Geometry: final body of the model. Coordinates: model frame, mm. Face numbers are marked on the shaded views. A direction names the side the tool comes from. Give positions to 0.01 mm unless a question says otherwise; leave off trailing zeros. Order: outer loops, then holes, each group sorted by start corner. A loop starts at its lowest first (then second) coordinate and runs counter-clockwise, first axis right, second up. Notation, with made-up numbers: (37.5, 76) - (82.5, 76) arc R25 cw to (82.5, 109) - close; hole circle Ø9 at (7.5, -4.75). An arc over 180 degrees is marked (long way). Use one line per item in the form item = value.
from build123d import *
from OCP.BRepFilletAPI import BRepFilletAPI_MakeChamfer

# Parameters (mm, degrees)
SKETCH1_W           = 12.7
SKETCH1_H           = 16
BOSS_EXTRUDE1_DEPTH = 22
SKETCH2_R           = 2.75
CUT_EXTRUDE1_DEPTH  = 239.308352823
SKETCH5_W           = 168.195
SKETCH5_H           = 59.75
CUT_EXTRUDE3_DEPTH  = 8
CHAMFER1_SIZE       = 10
CHAMFER1_SIZE2      = 5.773502692
SKETCH7_R           = 5.25
CUT_EXTRUDE4_DEPTH  = 10
CHAMFER2_SIZE       = 12


with BuildPart() as part:
    # Sketch1 → Boss-Extrude1 (new body)
    with BuildSketch(Plane.XY):
        Polygon((-12, 31.75), (200.195, 31.75), (233.895, 31.75), (233.895, -40), (200.895, -40), (-12.7, -40), (-45.7, -40), (-45.7, 31.75), align=None)
        with Locations((-6.35, -4.125)):
            Rectangle(SKETCH1_W, SKETCH1_H, mode=Mode.SUBTRACT)
        with Locations((194.545, -4.125)):
            Rectangle(SKETCH1_W, SKETCH1_H, mode=Mode.SUBTRACT)
    extrude(amount=BOSS_EXTRUDE1_DEPTH)

    # Sketch2 → Cut-Extrude1 (cut, through all)
    with BuildSketch(Plane.XY.offset(22)):
        with Locations((-6.35, 19.75)):
            Circle(SKETCH2_R)
        with Locations((-6.35, -28)):
            Circle(SKETCH2_R)
        with Locations(Location((194.545, -28, 0), (0, 0, 180))):
            Circle(SKETCH2_R)
        with Locations(Location((194.545, 19.75, 0), (0, 0, 180))):
            Circle(SKETCH2_R)
    extrude(amount=-CUT_EXTRUDE1_DEPTH, mode=Mode.SUBTRACT)

    # Sketch5 → Cut-Extrude3 (cut)
    with BuildSketch(Plane(origin=(0, 0, 0), x_dir=(-1, 0, 0), z_dir=(0, 0, -1))):
        with Locations((-94.0975, -10.125)):
            Rectangle(SKETCH5_W, SKETCH5_H)
    extrude(amount=-CUT_EXTRUDE3_DEPTH, mode=Mode.SUBTRACT)

    # Chamfer1: one chamfer whose edges measure the first distance from different faces: ONE call of the kernel's chamfer builder (chamfer() names one face for all edges)
    chamfer1_edges_1 = [part.edges().sort_by_distance(p)[0] for p in [
        (94.0975, -40, 22),
    ]]
    chamfer1_side_1 = [part.faces().sort_by_distance(p)[0] for p in [
        (94.0975, -40, 12.960016897),
    ]]
    chamfer1_edges_2 = [part.edges().sort_by_distance(p)[0] for p in [
        (94.0975, 31.75, 22),
    ]]
    chamfer1_side_2 = [part.faces().sort_by_distance(p)[0] for p in [
        (94.0975, 31.75, 11),
    ]]
    chamfer1 = BRepFilletAPI_MakeChamfer(part.part.solid().wrapped)
    for e in chamfer1_edges_1:
        chamfer1.Add(CHAMFER1_SIZE, CHAMFER1_SIZE2, e.wrapped, chamfer1_side_1[0].wrapped)  # the first distance lies on this face
    for e in chamfer1_edges_2:
        chamfer1.Add(CHAMFER1_SIZE, CHAMFER1_SIZE2, e.wrapped, chamfer1_side_2[0].wrapped)  # the first distance lies on this face
    add(Compound.cast(chamfer1.Shape()), mode=Mode.REPLACE)

    # Sketch7 → Cut-Extrude4 (cut)
    with BuildSketch(Plane.XY.offset(22)):
        with Locations((-6.35, 19.75)):
            Circle(SKETCH7_R)
        with Locations((-6.35, -28)):
            Circle(SKETCH7_R)
        with Locations((194.545, 19.75)):
            Circle(SKETCH7_R)
        with Locations((194.545, -28)):
            Circle(SKETCH7_R)
    extrude(amount=-CUT_EXTRUDE4_DEPTH, mode=Mode.SUBTRACT)

    # Chamfer2
    chamfer2_edges = [part.edges().sort_by_distance(p)[0] for p in [
        (-45.7, -4.125, 22),
        (233.895, -4.125, 22),
    ]]
    chamfer(chamfer2_edges, length=CHAMFER2_SIZE)


solid = part.part
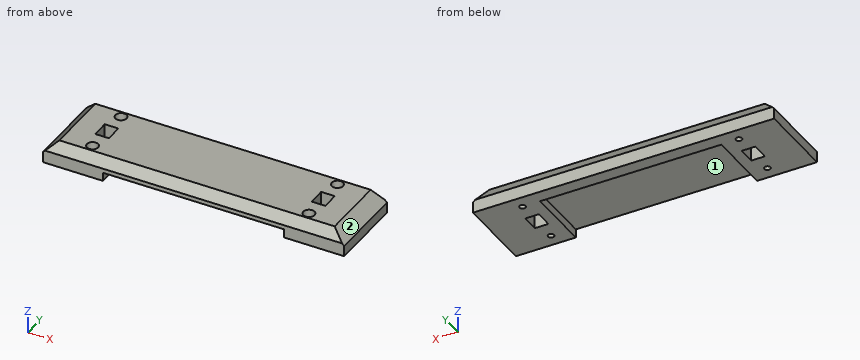
(1) Cut plane D-D on z = 5. Output: boundary loops of the cut face in (x, y) (3 decimals).
Computed values:
outline = (-45.7, -40) - (10, -40) - (10, 19.75) - (178.195, 19.75) - (178.195, -40) - (233.895, -40) - (233.895, 31.75) - (-45.7, 31.75) - close; hole (-12.7, -12.125) - (0, -12.125) - (0, 3.875) - (-12.7, 3.875) - close; hole circle Ø5.5 at (-6.35, -28); hole circle Ø5.5 at (-6.35, 19.75); hole (188.195, -12.125) - (200.895, -12.125) - (200.895, 3.875) - (188.195, 3.875) - close; hole circle Ø5.5 at (194.545, -28); hole circle Ø5.5 at (194.545, 19.75)
(2) Reachability of the marked faces 1 and 2 from +Z, -Z, +X, -X, +Y, -Y: full face, straight path, thin tool, end or side. Return the list, or none.
Computed values:
face_1 = -Z, -Y
face_2 = +Z, +X, +Y, -Y
(3) Cut plane B-B on x = 170. Output: boundary loops of the cut face in (y, z), plus the area to 3 significant figures.
Computed values:
outline = (-40, 8) - (19.75, 8) - (19.75, 0) - (31.75, 0) - (31.75, 12) - (25.98, 22) - (-34.23, 22) - (-40, 12) - close
area = 1,040 mm²
(4) Cut plane C-C on x = -6.35. Give the number of separate pieces and of enclosed holes in the cut face, plus the area to 3 significant figures.
Computed values:
separate_pieces = 4
enclosed_holes = 0
area = 827 mm²
(5) Contact query for flat-ended pins moving along their axis: pin 1 Ø4 at (x, y) = (126, -14) entering from -Z; pin 2 Ø6 at (x, z) = (96, 18.5) entering from -Y; pin 3 Ø8.5 at (x, y) = (194.545, -28) entering from +Z. Output: stop coordinate, or through.
Computed values:
pin_1 = 8
pin_2 = -37.98
pin_3 = 12
(6) Cut plane A-A on y = 1.5. Output: boundary loops of the cut face in (x, z) (3 decimals).
Computed values:
outline = (-45.7, 0) - (-12.7, 0) - (-12.7, 22) - (-33.7, 22) - (-45.7, 10) - close; (0, 0) - (10, 0) - (10, 8) - (178.195, 8) - (178.195, 0) - (188.195, 0) - (188.195, 22) - (0, 22) - close; (200.895, 0) - (233.895, 0) - (233.895, 10) - (221.895, 22) - (200.895, 22) - close
(7) Ray query, line 1 along X through (y, z) = (3, 1.5) (3 decimals); line 2 along X through (y, z) = (15.5, 4) (3 decimals); line 3 along Z through (x, y) = (16, 7). Return the intervals inside material, ascending.
Computed values:
line_1 = -45.7 to -12.7, 0 to 10, 178.195 to 188.195, 200.895 to 233.895
line_2 = -45.7 to 10, 178.195 to 233.895
line_3 = 8 to 22
